Source: CAD feature listing. Evaluate the final solid. Frame: model axes, mm. A direction names the side the tool comes from. Give positions to 0.01 mm unless a question says otherwise; leave off trailing zeros. Order: outer loops, then holes, each group sorted by start corner. A loop starts at its lowest first (then second) coordinate and runs counter-clockwise, first axis right, second up. Notation, with made-up numbers: M 55.25,-30.5 L 97.25,-30.5 A5 cw 97.25,-23.5 Z; hole C 42,7.25 d5. An arc over 180 degrees is marked long. Answer in a Markdown table with one row per item. Add a question column.
(1) Section query D-D, the plane x = 321. Return loops of the section in (y, z), plus the area to 3 significant figures.
(2) Section query B-B, the plane x = 381. Return loops of the section in (y, z).
(3) Section query A-A, the plane y = -5.25. Return loops of the section in (x, z), plus the area to 3 significant figures.
(4) Section query C-C, the plane z = 482.5. Return loops of the section in (x, y).
(5) Material intervals for line 1 along Z through (x, y) = (386, -4.25); line 2 along Z through (x, y) = (626, -5); line 3 along X through (y, z) = (-3.75, 411), sorted ascending.
(6) Pin query (flat end, axial travel): P1, Ø1, axis at x = 442.5, z = 157.5, coming from the -Y side; P2, Ø6, axis at x = 445, z = 283.5, coming from the +Y side; P3, Ø10, axis at x = 477, z = 11.5, coming from the -Y side. Return the tip coordinate at first contact, or that it passes through.
(7) Set-up query: faces 4 (the face through (460, 0, -115.008)), 5 (the face through (460, -5, 5.642)), 6 (the face through (460, 9.398, 220)). Return all of +Z, -Z, +X, -X, +Y, -Y with unobstructed straight access to the full face (end or side cutting, diameter ignored); none if empty.
(8) Mould query, pull axis X, two halves, no side actions, for faces 1 (the face through (460, 0, 12)), 2 (the face through (257.955, 0, 220)), 3 (the face through (667.53, 0, 211)). Classes: pulls with the +X half, pulls with the -X half, needs draft (parallel to the pull), parting line crosses it, or undercut.
from build123d import *

# Parameters (mm, degrees)
F1_DEPTH      = 12.7
F1_DEPTH_BACK = 12.7
F0_W          = 371.475
F0_H          = 622.3
F2_DEPTH      = 9.398
F2_DEPTH_BACK = 9.398
F3_W          = 193.675
F3_H          = 330.2
F4_DEPTH      = 12.7


# Not quite as in the source:
# - a feature names something its author has since deleted; it is built from what else it names


with BuildPart() as f1:
    # F0 (on Front) → F1 (new body, two sides)
    with BuildSketch(Plane.XZ) as f1_sk:
        Polygon((277.0045676708, 526.3417813361), (648.4795676708, 526.3417813361), (667.5295676708, 545.3917813361), (257.9545676708, 545.3917813361), align=None)
        Polygon((277.0045676708, -95.9582186639), (277.0045676708, 526.3417813361), (257.9545676708, 545.3917813361), (257.9545676708, -115.0082186639), align=None)
        Polygon((667.5295676708, 545.3917813361), (648.4795676708, 526.3417813361), (648.4795676708, -95.9582186639), (667.5295676708, -115.0082186639), align=None)
        Polygon((667.5295676708, -115.0082186639), (648.4795676708, -95.9582186639), (277.0045676708, -95.9582186639), (257.9545676708, -115.0082186639), align=None)
    extrude(amount=-F1_DEPTH)
    extrude(f1_sk.sketch, amount=F1_DEPTH_BACK)

    # F0 (on Front) → F2 (join, two sides)
    with BuildSketch(Plane.XZ) as f2_sk:
        Polygon((667.5295676708, 545.3917813361), (648.4795676708, 526.3417813361), (648.4795676708, -95.9582186639), (667.5295676708, -115.0082186639), align=None)
        Polygon((277.0045676708, 526.3417813361), (648.4795676708, 526.3417813361), (667.5295676708, 545.3917813361), (257.9545676708, 545.3917813361), align=None)
        Polygon((667.5295676708, -115.0082186639), (648.4795676708, -95.9582186639), (277.0045676708, -95.9582186639), (257.9545676708, -115.0082186639), align=None)
        Polygon((277.0045676708, -95.9582186639), (277.0045676708, 526.3417813361), (257.9545676708, 545.3917813361), (257.9545676708, -115.0082186639), align=None)
        with Locations((462.7420676708, 215.1917813361)):
            Rectangle(F0_W, F0_H)
    extrude(amount=F2_DEPTH)
    extrude(f2_sk.sketch, amount=-F2_DEPTH_BACK)

    # F3 (on face) → F4 (cut)
    with BuildSketch(Plane.XZ):
        Polygon((276.66666205, 5.6417813361), (648.4795676708, 5.6417813361), (648.4795676708, 18.3417813361), (277.0045676708, 18.3417813361), align=None)
        Polygon((572.2795676708, 456.4917813361), (572.2795676708, 469.1917813361), (353.2045676708, 469.1917813361), (353.2045676708, 456.4917813361), (353.2045676708, 126.2917813361), (277.0045676708, 126.2917813361), (277.0045676708, 113.5917813361), (648.4795676708, 113.5917813361), (648.4795676708, 126.2917813361), (572.2795676708, 126.2917813361), align=None)
        with Locations((462.7420676708, 291.3917813361)):
            Rectangle(F3_W, F3_H, mode=Mode.SUBTRACT)
    extrude(amount=F4_DEPTH, mode=Mode.SUBTRACT)


solid = f1.part
Values follow:
| question | item | result |
|---|---|---|
| 1 | outline | M -12.7,-115.01 L 12.7,-115.01 L 12.7,-95.96 L 9.4,-95.96 L 9.4,526.34 L 12.7,526.34 L 12.7,545.39 L -12.7,545.39 L -12.7,526.34 L -9.4,526.34 L -9.4,126.29 L 0,126.29 L 0,113.59 L -9.4,113.59 L -9.4,18.34 L 0,18.34 L 0,5.64 L -9.4,5.64 L -9.4,-95.96 L -12.7,-95.96 Z |
| 1 | area | 12,400 mm² |
| 2 | outline | M -12.7,-115.01 L 12.7,-115.01 L 12.7,-95.96 L 9.4,-95.96 L 9.4,526.34 L 12.7,526.34 L 12.7,545.39 L -12.7,545.39 L -12.7,526.34 L -9.4,526.34 L -9.4,469.19 L 0,469.19 L 0,456.49 L -9.4,456.49 L -9.4,126.29 L 0,126.29 L 0,113.59 L -9.4,113.59 L -9.4,18.34 L 0,18.34 L 0,5.64 L -9.4,5.64 L -9.4,-95.96 L -12.7,-95.96 Z |
| 3 | outline | M 257.95,-115.01 L 667.53,-115.01 L 667.53,545.39 L 257.95,545.39 Z; M 365.9,126.29 L 559.58,126.29 L 559.58,456.49 L 365.9,456.49 Z; hole M 276.67,5.64 L 648.48,5.64 L 648.48,18.34 L 277,18.34 Z; hole M 277,113.59 L 648.48,113.59 L 648.48,126.29 L 572.28,126.29 L 572.28,469.19 L 353.2,469.19 L 353.2,126.29 L 277,126.29 Z |
| 3 | area | 250,000 mm² |
| 4 | outline | M 257.95,-12.7 L 277,-12.7 L 277,-9.4 L 648.48,-9.4 L 648.48,-12.7 L 667.53,-12.7 L 667.53,12.7 L 648.48,12.7 L 648.48,9.4 L 277,9.4 L 277,12.7 L 257.95,12.7 Z |
| 5 | line 1 | z = -115.01 to 5.64, 18.34 to 113.59, 126.29 to 456.49, 469.19 to 545.39 |
| 5 | line 2 | z = -115.01 to 5.64, 18.34 to 113.59, 126.29 to 545.39 |
| 5 | line 3 | x = 257.95 to 353.2, 365.9 to 559.58, 572.28 to 667.53 |
| 6 | P1 | stops at y = -9.4 |
| 6 | P2 | stops at y = 9.4 |
| 6 | P3 | stops at y = 0 |
| 7 | face 4 | -Z, +X, -X, +Y, -Y |
| 7 | face 5 | -Y |
| 7 | face 6 | +Y |
| 8 | face 1 | undercut |
| 8 | face 2 | pulls with the -X half |
| 8 | face 3 | pulls with the +X half |
